from build123d import *

# Parameters (mm, degrees)
SKETCH1_R           = 25
SKETCH1_R_2         = 22.5
BOSS_EXTRUDE1_DEPTH = 280


with BuildPart() as part:
    # Sketch1 → Boss-Extrude1 (new body)
    with BuildSketch(Plane(origin=(0, 0, 0), x_dir=(1, 0, 0), z_dir=(0, 1, 0))):
        Circle(SKETCH1_R)
        Circle(SKETCH1_R_2, mode=Mode.SUBTRACT)
    extrude(amount=BOSS_EXTRUDE1_DEPTH)

    # Sketch2 → Cut-Revolve1 (revolve, cut)
    with BuildSketch(Plane.XY):
        Polygon((24, 275), (22.5, 275), (22.157069883, 275), (22.157069883, 277), (22.5, 277), (24, 277), align=None)
        Polygon((22.5, 8), (24, 8), (24, 10), (21.749142676, 10), (21.749142676, 8), align=None)
        Polygon((25, 3), (24, 3), (24, 5), (25.376612155, 5), (25.376612155, 3), align=None)
    revolve(axis=Axis((0, 307.21500467, 0), (0, -1, 0)), mode=Mode.SUBTRACT)


solid = part.part
For this review, take the finished solid that the model builds, in its own axes (mm). A direction names the side the tool comes from. Round coordinates to 2 decimals unless told otherwise and drop trailing zeros. Write each loop counter-clockwise with the first axis right and the second up, starting at its lowest first coordinate (ties: lowest second). Pieces come first, ordered by that corner, then holes. Notation, with made-up numbers: (-19, 36) -> (2, 36) arc R22 ccw to (2, 47) -> close; hole circle Ø4 at (42.25, 52). An arc over 180 degrees is marked (long way). Use CSV: the item, a comma, the result in double quotes.
(1) To check wall thickness, follow L1, parallel to Z at x = 0, y = 275.9; L2, parallel to Z at x = 0, y = 277.85. State the ranges of each line that lie inside material, in increasing order. Write a range as [from, to].
Computed values:
L1,"[-25, -24], [24, 25]"
L2,"[-25, -22.5], [22.5, 25]"
(2) Draft analysis for pull direction Z (two halves, no side actions). For faces 1 (the face through (-22.34, 0, -3.82)), 2 (the face through (-23.977, 4.014, 1.055)), 3 (the face through (10.382, 140.645, 19.961)), 4 (the face through (-23.977, 9.014, 1.055)), state which applies: +Z half, -Z half, draft (parallel to the pull), parting line (faces both ways), or undercut.
Computed values:
face 1,"draft"
face 2,"parting line"
face 3,"undercut"
face 4,"undercut"
(3) Consider section C-C, the plane y = 23.5. Give the boundary of the cut face in (x, z).
Computed values:
outline,"circle Ø50 at (0, 0); hole circle Ø45 at (0, 0)"
(4) Clearance check with flat-ended pins moving along their axes: P1, Ø25, axis at x = -8, z = -2, coming from the -Y side; P2, Ø10, axis at x = 18, y = 247.5, coming from the -Z side; P3, Ø6, axis at y = 72.5, z = -7.5, coming from the +X side; P4, Ø2, axis at y = 89.5, z = -9, coming from the +X side. State where each tip first meets the part, or that it passes through.
Computed values:
P1,"through"
P2,"z = -21.35"
P3,"x = 24.59"
P4,"x = 23.69"
(5) For faces 5 (the face through (23.846, 1.479, -7.509)), 6 (the face through (9.4, 3, 22.3)), list the 3-axis set-ups (+Z, -Z, +X, -X, +Y, -Y) from which the entire face can be reached by the end or side of a thin tool; tool diameter is ignored.
Computed values:
face 5,"+Y, -Y"
face 6,"none"
